Verification items for the finished model (mm, model axes). A direction names the side the tool comes from. Give positions to 0.01 mm unless a question says otherwise; leave off trailing zeros. Loops run counter-clockwise (first coordinate to the right, second up) from the corner with the lowest first, then second, coordinate; pieces in that order, holes last. Notation, with made-up numbers: M 66.25,-3.75 L 87.25,-3.75 A3 ccw 87.25,1.25 Z; hole C 83,-9 d5. An arc over 180 degrees is marked long. Use a Markdown table: item, result.
from build123d import *

# Parameters (mm, degrees)
F0_W     = 19.05
F0_H     = 19.05
F1_DEPTH = 6.35
F2_R     = 1.27
F3_DEPTH = 25.4


with BuildPart() as f1:
    # F0 (on Front) → F1 (new body)
    with BuildSketch(Plane.XZ):
        Polygon((-10.8805632712, 62.4568768001), (-10.8805632712, 24.3568768001), (8.1694367288, 24.3568768001), (8.1694367288, 43.4068768001), (46.2694367288, 43.4068768001), (46.2694367288, 62.4568768001), align=None)
        with Locations((-1.3555632712, 14.8318768001)):
            Rectangle(F0_W, F0_H)
        Polygon((8.1694367288, 24.3568768001), (8.1694367288, 5.3068768001), (27.2194367288, 5.3068768001), (27.2194367288, -32.7931231999), (46.2694367288, -32.7931231999), (46.2694367288, 24.3568768001), align=None)
        Polygon((8.1694367288, 5.3068768001), (-10.8805632712, 5.3068768001), (-10.8805632712, -13.7431231999), (-48.9805632712, -13.7431231999), (-48.9805632712, -32.7931231999), (8.1694367288, -32.7931231999), align=None)
        Polygon((-29.9305632712, 62.4568768001), (-48.9805632712, 62.4568768001), (-48.9805632712, 5.3068768001), (-10.8805632712, 5.3068768001), (-10.8805632712, 24.3568768001), (-29.9305632712, 24.3568768001), align=None)
    extrude(amount=F1_DEPTH)

    # F2 (on face) → F3 (cut)
    with BuildSketch(Plane.XZ.offset(6.35)):
        with Locations((-46.6758534312, 59.7021207213)):
            Circle(F2_R)
    extrude(amount=-F3_DEPTH, mode=Mode.SUBTRACT)


solid = f1.part
(1) Cross-section at B-B on z = 52. Record the cut outline in (x, y), then the cut area to 3 significant figures.
Results below:
| item | result |
|---|---|
| outline | M -48.98,-6.35 L -29.93,-6.35 L -29.93,0 L -48.98,0 Z; M -10.88,-6.35 L 46.27,-6.35 L 46.27,0 L -10.88,0 Z |
| area | 484 mm^2 |
(2) Cross-section at A-A on x = -23.5. Record the cut outline in (y, z).
Results below:
| item | result |
|---|---|
| outline | M -6.35,-32.79 L 0,-32.79 L 0,-13.74 L -6.35,-13.74 Z; M -6.35,5.31 L 0,5.31 L 0,24.36 L -6.35,24.36 Z |
(3) Material ranges on line 1 (X direction, y = -2.75, z = -6.5); line 2 (X direction, y = -2.5, z = 34); line 3 (Z direction, x = -43, y = -5.25), recorded low to high.
Results below:
| item | result |
|---|---|
| line 1 | -10.88 to 8.17, 27.22 to 46.27 |
| line 2 | -48.98 to -29.93, -10.88 to 8.17 |
| line 3 | -32.79 to -13.74, 5.31 to 62.46 |
(4) Set-up check for faces 1 (the flat face through (-10.881, -3, 44)), 2 (the flat face through (27, -3, 43.407)), 3 (the flat face through (18, -3, 5.307)), 4 (the flat face through (-30, -3, 5.307)): record each of +Z, -Z, +X, -X, +Y, -Y from which the full face is reachable in a straight line by a thin tool's end or side.
Results below:
| item | result |
|---|---|
| face 1 | +Z, +Y, -Y |
| face 2 | +X, +Y, -Y |
| face 3 | -Z, +Y, -Y |
| face 4 | -X, +Y, -Y |
(5) Cross-section at C-C on y = -5. Record the cut outline in (x, z), then the cut area to 3 significant figures.
Results below:
| item | result |
|---|---|
| outline | M -48.98,-32.79 L 8.17,-32.79 L 8.17,5.31 L 27.22,5.31 L 27.22,-32.79 L 46.27,-32.79 L 46.27,24.36 L 8.17,24.36 L 8.17,43.41 L 46.27,43.41 L 46.27,62.46 L -10.88,62.46 L -10.88,24.36 L -29.93,24.36 L -29.93,62.46 L -48.98,62.46 L -48.98,5.31 L -10.88,5.31 L -10.88,-13.74 L -48.98,-13.74 Z; hole C -46.68,59.7 d2.54 |
| area | 6,160 mm^2 |
(6) Gauge pin test, flat ends, axial feed: P1, Ø1.9, axis at y = -3.5, z = -5, coming from the -X side; P2, Ø1.9, axis at y = -3, z = 32.5, coming from the +X side; P3, Ø2, axis at x = -46.68, z = 59.7, coming from the +Y side. Record the tip position at first contact, or that the pin passes through.
Results below:
| item | result |
|---|---|
| P1 | x = -10.88 |
| P2 | x = 8.17 |
| P3 | through |
